from build123d import *

# Parameters (mm, degrees)
SKETCH051_W  = 300
SKETCH051_H  = 60
PAD010_DEPTH = 200
SKETCH052_W  = 312
SKETCH052_H  = 50
PAD011_DEPTH = 206
SKETCH053_W  = 412
SKETCH053_H  = 512
PAD012_DEPTH = 6


with BuildPart() as body008:
    # Sketch051 → Pad010 (new body, symmetric)
    with BuildSketch(Plane.XZ):
        with Locations((0, 30)):
            Rectangle(SKETCH051_W, SKETCH051_H)
    extrude(amount=PAD010_DEPTH, both=True)


with BuildPart() as cut006:
    # Sketch052 → Pad011 (new body, symmetric)
    with BuildSketch(Plane.XZ):
        with Locations((0, 25)):
            Rectangle(SKETCH052_W, SKETCH052_H)
    extrude(amount=PAD011_DEPTH, both=True)

    # Sketch053 (on Face3 of Pad011) → Pad012 (join)
    with BuildSketch(Plane(origin=(0, 0, 50), x_dir=(-1, 0, 0), z_dir=(0, 0, 1))):
        Rectangle(SKETCH053_W, SKETCH053_H)
    extrude(amount=PAD012_DEPTH)

    # Cut006: cut Body008
    add(body008.part, mode=Mode.SUBTRACT)


solid = cut006.part
Part model, mm, in its own coordinate system. A direction names the side the tool comes from. Coordinates: 2 decimals unless noted, no trailing zeros. Order: outer loops, then holes, each group sorted by start corner. A loop starts at its lowest first (then second) coordinate and runs counter-clockwise, first axis right, second up. Notation, with made-up numbers: (77, 22.5) - (102, 22.5) arc R8 ccw to (102, 31.5) - close; hole circle Ø10 at (-14.75, 78.25). An arc over 180 degrees is marked (long way). Use CSV: the item, a comma, the result in double quotes.
Item 1: Saw through at A-A on z = 7.5. Give the cut face in (x, y), and give its area (3 significant figures).
Solved:
outline,"(-156, -206) - (156, -206) - (156, 206) - (-156, 206) - close; hole (-150, -200) - (150, -200) - (150, 200) - (-150, 200) - close"
area,"8,540 mm²"
Item 2: Mould opens along Y. For faces 6 (the face through (-2, 206, 25)), 7 (the face through (-150, -3, 28)), 8 (the face through (150, -3, 28)), 9 (the face through (-180, -4, 56)) say: +Y half, -Y half, draft (parallel to the pull), parting line (faces both ways), or undercut.
Solved:
face 6,"+Y half"
face 7,"undercut"
face 8,"undercut"
face 9,"draft"
Item 3: 3-axis set-ups, long thin cutter, end or side, ignore diameter. For faces 1 (the face through (-2, -206, 25)), 2 (the face through (-156, -3, 25)), 3 (the face through (156, -3, 25)), 4 (the face through (-2, -200, 28)), 5 (the face through (-151, -1, 0)): which of +Z, -Z, +X, -X, +Y, -Y reach the whole face in a straight line?
Solved:
face 1,"-Z, +X, -X, -Y"
face 2,"-Z, -X, +Y, -Y"
face 3,"-Z, +X, +Y, -Y"
face 4,"+Z, -Z"
face 5,"-Z, +X, -X, +Y, -Y"
Item 4: Saw through at D-D on x = 178.5. Give the cut face in (y, z).
Solved:
outline,"(-256, 50) - (256, 50) - (256, 56) - (-256, 56) - close"
Item 5: Saw through at B-B on x = -77.5. Give the cut face in (y, z), and give its area (3 significant figures).
Solved:
outline,"(-256, 50) - (-206, 50) - (-206, 0) - (-200, 0) - (-200, 56) - (-256, 56) - close; (200, 0) - (206, 0) - (206, 50) - (256, 50) - (256, 56) - (200, 56) - close"
area,"1,270 mm²"
Item 6: Probe probe 1 along Y at (x, z) = (55.5, 6.5); probe 2 along X at (y, z) = (-80.5, 23); probe 3 along Z at (x, y) = (129, -230). List the from-to ranges inside material, lowest first.
Solved:
probe 1,"y = -206 to -200, 200 to 206"
probe 2,"x = -156 to -150, 150 to 156"
probe 3,"z = 50 to 56"
Item 7: Saw through at C-C on y = 153. Give the cut face in (x, z), and give its area (3 significant figures).
Solved:
outline,"(-206, 50) - (-156, 50) - (-156, 0) - (-150, 0) - (-150, 56) - (-206, 56) - close; (150, 0) - (156, 0) - (156, 50) - (206, 50) - (206, 56) - (150, 56) - close"
area,"1,270 mm²"
Item 8: Drop flat-ended pins along their axis: P1, Ø6, axis at x = 11.5, z = 15, coming from the +Y side; P2, Ø8, axis at x = 102.5, z = 41.5, coming from the -Y side; P3, Ø4, axis at y = 36.5, z = 26, coming from the -X side. Give the stop position or say it passes through.
Solved:
P1,"stops at y = 206"
P2,"stops at y = -206"
P3,"stops at x = -156"
